The model under review builds one solid part; all positions refer to its coordinate system, in mm. Give positions to 0.01 mm unless a question says otherwise; leave off trailing zeros. Order: outer loops, then holes, each group sorted by start corner. A loop starts at its lowest first (then second) coordinate and runs counter-clockwise, first axis right, second up.
```python
from build123d import *

# Parameters (mm, degrees)
SKETCH1_R           = 2.6
BOSS_EXTRUDE3_DEPTH = 10
SKETCH5_R           = 5
CUT_EXTRUDE3_DEPTH  = 20
CHAMFER1_SIZE       = 1


with BuildPart() as part:
    # Sketch1 → Boss-Extrude3 (new body)
    with BuildSketch(Plane(origin=(0, 0, 0), x_dir=(1, 0, 0), z_dir=(0, 1, 0))):
        with BuildLine():
            Line((-13.5, -10), (13.5, -10))
            ThreePointArc((13.5, -10), (15.621320344, -9.121320344), (16.5, -7))
            Line((16.5, -7), (16.5, 7))
            ThreePointArc((16.5, 7), (15.621320344, 9.121320344), (13.5, 10))
            Line((13.5, 10), (-13.5, 10))
            ThreePointArc((-13.5, 10), (-15.621320344, 9.121320344), (-16.5, 7))
            Line((-16.5, 7), (-16.5, -7))
            ThreePointArc((-16.5, -7), (-15.621320344, -9.121320344), (-13.5, -10))
        make_face()
        with Locations(Location((10.5, 0, 0), (0, 0, 270))):
            Circle(SKETCH1_R, mode=Mode.SUBTRACT)
        with Locations(Location((-10.5, 0, 0), (0, 0, 90))):
            Circle(SKETCH1_R, mode=Mode.SUBTRACT)
    extrude(amount=BOSS_EXTRUDE3_DEPTH)

    # Sketch5 → Cut-Extrude3 (cut)
    with BuildSketch(Plane(origin=(0, 0, -10), x_dir=(-1, 0, 0), z_dir=(0, 0, -1))):
        with Locations((0, 10.2)):
            Circle(SKETCH5_R)
    extrude(amount=-CUT_EXTRUDE3_DEPTH, mode=Mode.SUBTRACT)

    # Chamfer1
    chamfer1_edges = [part.edges().sort_by_distance(p)[0] for p in [
        (0, 0, 10),
        (-15.621320344, 0, 9.121320344),
        (-16.5, 0, 0),
        (-15.621320344, 0, -9.121320344),
        (0, 0, -10),
        (15.621320344, 0, -9.121320344),
        (16.5, 0, 0),
        (15.621320344, 0, 9.121320344),
    ]]
    chamfer(chamfer1_edges, length=CHAMFER1_SIZE)


solid = part.part
```
1. Take a section at D-D (y = 6.75). Write out the cut boundary in (x, z).
2. Take a section at A-A (y = 2). Write out the cut boundary in (x, z).
3. Insertion check: pin 1 (4.5 mm diameter, centred on x = -10.5, z = 0, fed in from -Y). The pin has a flat end and moves straight along its axis. Give the tip position at first contact, or say it passes through.
4. Take a section at C-C (x = -10.5). Write out the cut boundary in (y, z).
5. Draft analysis for pull direction X (two halves, no side actions). For faces 1 (the flat face through (0.2, 0.5, -9.5)), 2 (the cylindrical face through (7.96, 4.93, -0.56)), 3 (the conical face through (-15.203, 0.382, 8.666)), state which applies: pulls with the +X half, pulls with the -X half, needs draft (parallel to the pull), parting line crosses it, or undercut.
6. To check wall thickness, follow line 1 (X direction, y = 4.5, z = 0); line 2 (Z direction, x = -10.5, y = 5.5); line 3 (X direction, y = 2.25, z = 2). State the ranges of each line that lie inside material, in increasing order.
Answer:
1. outline: (-16.5, -7) arc R3 ccw to (-13.5, -10) - (-3.62, -10) - (-3.62, 10) - (-13.5, 10) arc R3 ccw to (-16.5, 7) - close; (3.62, -10) - (13.5, -10) arc R3 ccw to (16.5, -7) - (16.5, 7) arc R3 ccw to (13.5, 10) - (3.62, 10) - close; hole circle Ø5.2 at (-10.5, 0); hole circle Ø5.2 at (10.5, 0)
2. outline: (-16.5, -7) arc R3 ccw to (-13.5, -10) - (13.5, -10) arc R3 ccw to (16.5, -7) - (16.5, 7) arc R3 ccw to (13.5, 10) - (-13.5, 10) arc R3 ccw to (-16.5, 7) - close; hole circle Ø5.2 at (-10.5, 0); hole circle Ø5.2 at (10.5, 0)
3. pin 1: passes through
4. outline: (0, -9) - (1, -10) - (10, -10) - (10, -2.6) - (0, -2.6) - close; (0, 2.6) - (10, 2.6) - (10, 10) - (1, 10) - (0, 9) - close
5. face 1: needs draft
5. face 2: undercut
5. face 3: pulls with the -X half
6. line 1: x = -16.5 to -13.1, -7.9 to 7.9, 13.1 to 16.5
6. line 2: z = -10 to -2.6, 2.6 to 10
6. line 3: x = -16.5 to -12.16, -8.84 to 8.84, 12.16 to 16.5
